For this review, take the finished solid that the model builds, in its own axes (mm). Face numbers are marked on the shaded views. A direction names the side the tool comes from. Coordinates: 2 decimals unless noted, no trailing zeros. Write each loop counter-clockwise with the first axis right and the second up, starting at its lowest first coordinate (ties: lowest second). Pieces come first, ordered by that corner, then holes.
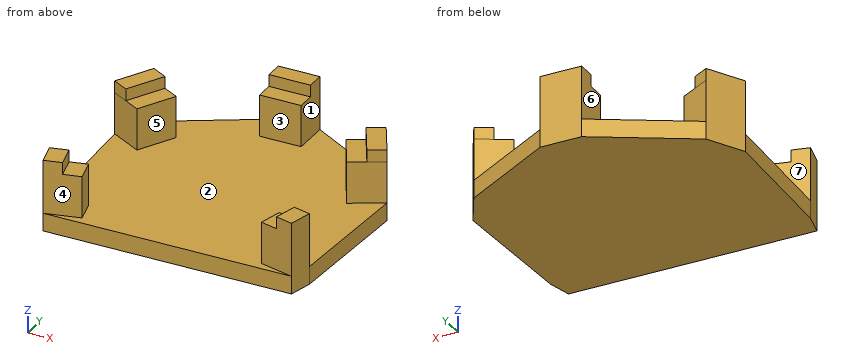
```python
from build123d import *

# Parameters (mm, degrees)
SKETCH2_W             = 7
SKETCH2_H             = 3
BOSS_EXTRUDE1_DEPTH   = 2
BOSS_EXTRUDE1_2_DEPTH = 2
BOSS_EXTRUDE1_3_DEPTH = 2
BOSS_EXTRUDE1_4_DEPTH = 2
BOSS_EXTRUDE1_5_DEPTH = 2
SKETCH3_W             = 7
SKETCH3_H             = 6
BOSS_EXTRUDE2_DEPTH   = 7
BOSS_EXTRUDE3_DEPTH   = 3


with BuildPart() as part:
    # Sketch2 → Boss-Extrude1 (new body)
    with BuildSketch(Plane.XY):
        with Locations((0, 28.5)):
            Rectangle(SKETCH2_W, SKETCH2_H)
    extrude(amount=BOSS_EXTRUDE1_DEPTH)



with BuildPart() as body_2:
    # Sketch2 → Boss-Extrude1 2 (new body)
    with BuildSketch(Plane.XY):
        Polygon((-18.954098941, -7.515454311), (-18, -11.4), (-20.913409267, -12.115574206), (-21.867508208, -8.231028517), align=None)
    extrude(amount=BOSS_EXTRUDE1_2_DEPTH)


with BuildPart() as body_3:
    # Sketch2 → Boss-Extrude1 3 (new body)
    with BuildSketch(Plane.XY):
        Polygon((-20.286715624, 13.13324432), (-16.913284376, 19.26675568), (-19.541932102, 20.71251193), (-22.91536335, 14.579000569), align=None)
    extrude(amount=BOSS_EXTRUDE1_3_DEPTH)


with BuildPart() as body_4:
    # Sketch2 → Boss-Extrude1 4 (new body)
    with BuildSketch(Plane.XY):
        Polygon((22.91536335, 14.579000569), (19.541932102, 20.71251193), (16.913284376, 19.26675568), (20.286715624, 13.13324432), align=None)
    extrude(amount=BOSS_EXTRUDE1_4_DEPTH)


with BuildPart() as body_5:
    # Sketch2 → Boss-Extrude1 5 (new body)
    with BuildSketch(Plane.XY):
        Polygon((21.867508208, -8.231028517), (20.913409267, -12.115574206), (18, -11.4), (18.954098941, -7.515454311), align=None)
    extrude(amount=BOSS_EXTRUDE1_5_DEPTH)


with BuildPart() as part_1:
    add(part.part)

    add(body_2.part)  # Boss-Extrude2 merges body 2

    add(body_3.part)  # Boss-Extrude2 merges body 3

    add(body_4.part)  # Boss-Extrude2 merges body 4

    add(body_5.part)  # Boss-Extrude2 merges body 5
    # Sketch3 → Boss-Extrude2 (add)
    with BuildSketch(Plane.XY):
        Polygon((20.913409267, -12.115574206), (21.867508208, -8.231028517), (16.040689674, -6.799880105), (15.086590733, -10.684425794), align=None)
        Polygon((22.91536335, 14.579000569), (19.541932102, 20.71251193), (14.28463665, 17.820999431), (17.658067898, 11.68748807), align=None)
        with Locations((0, 27)):
            Rectangle(SKETCH3_W, SKETCH3_H)
        Polygon((-17.658067898, 11.68748807), (-14.28463665, 17.820999431), (-19.541932102, 20.71251193), (-22.91536335, 14.579000569), align=None)
        Polygon((-15.086590733, -10.684425794), (-16.040689674, -6.799880105), (-21.867508208, -8.231028517), (-20.913409267, -12.115574206), align=None)
    extrude(amount=-BOSS_EXTRUDE2_DEPTH)

    # Sketch4 → Boss-Extrude3 (add)
    with BuildSketch(Plane(origin=(0, 0, -7), x_dir=(-1, 0, 0), z_dir=(0, 0, -1))):
        Polygon((-21.867508208, -8.231028517), (-22.91536335, 14.579000569), (-19.541932102, 20.71251193), (-3.5, 30), (3.5, 30), (19.541932102, 20.71251193), (22.91536335, 14.579000569), (21.867508208, -8.231028517), (20.913409267, -12.115574206), (-20.913409267, -12.115574206), align=None)
    extrude(amount=BOSS_EXTRUDE3_DEPTH)


solid = part_1.part
```
Q1. Clearance check with flat-ended pins moving along their axes: pin 1 Ø4 at (y, z) = (12, -0.5) entering from +X; pin 2 Ø2 at (x, z) = (-0.5, -5) entering from -Y; pin 3 Ø4 at (x, z) = (14, -6) entering from +Y. State where each tip first meets the part, or that it passes through.
Ans:
pin 1: stops at x = 21.86
pin 2: stops at y = 24
pin 3: stops at y = 24.92
Q2. Add section C-C (x = -2). State the section outline as (y, z) points.
Ans:
outline: (-12.12, -10) - (30, -10) - (30, 2) - (27, 2) - (27, 0) - (24, 0) - (24, -7) - (-12.12, -7) - close
Q3. Draft analysis for pull direction Y (two halves, no side actions). For the marked faces 1, 2 and 3, state which applies: +Y half, -Y half, draft (parallel to the pull), parting line (faces both ways), or undercut.
Ans:
face 1: draft
face 2: undercut
face 3: -Y half
Q4. Tool access review of the marked faces 4, 5, 6 and 7: name each direction out of +Z, -Z, +X, -X, +Y, -Y from which nothing blocks a thin tool from reaching the whole face with its end or side.
Ans:
face 4: +Z, -Y
face 5: +Z
face 6: +Z, -X, +Y, -Y
face 7: +Z, -X
Q5. For probe 1 along Z at (x, y) = (14, -4); probe 2 along X at (y, z) = (15.5, -6.5); probe 3 along Y at (x, z) = (-19, 0.25), list the stretches that pass through material, from the lowest coordinate up.
Ans:
probe 1: z = -10 to -7
probe 2: x = -22.41 to -15.56, 15.56 to 22.41
probe 3: y = -11.65 to -7.53, 15.47 to 20.41
Q6. Add section A-A (z = -3.75). State the section outline as (x, y) points.
Ans:
outline: (-22.92, 14.58) - (-17.66, 11.69) - (-14.28, 17.82) - (-19.54, 20.71) - close; (-21.87, -8.23) - (-20.91, -12.12) - (-15.09, -10.68) - (-16.04, -6.8) - close; (-3.5, 24) - (3.5, 24) - (3.5, 30) - (-3.5, 30) - close; (14.28, 17.82) - (17.66, 11.69) - (22.92, 14.58) - (19.54, 20.71) - close; (15.09, -10.68) - (20.91, -12.12) - (21.87, -8.23) - (16.04, -6.8) - close
Q7. Add section D-D (y = -5). State the section outline as (x, z) points.
Ans:
outline: (-22.02, -10) - (22.02, -10) - (22.02, -7) - (-22.02, -7) - close
Q8. Add section B-B (z = -8.5). State the section outline as (x, y) points, then the cut area to 3 significant figures.
Ans:
outline: (-22.92, 14.58) - (-21.87, -8.23) - (-20.91, -12.12) - (20.91, -12.12) - (21.87, -8.23) - (22.92, 14.58) - (19.54, 20.71) - (3.5, 30) - (-3.5, 30) - (-19.54, 20.71) - close
area: 1,660 mm2
